from build123d import *

# Parameters (mm, degrees)
ESBO_O1_R                = 2.500003623
ESBO_O1_R_2              = 2.499998411
ESBO_O1_R_3              = 2.500000084
ESBO_O1_R_4              = 2.500000523
ESBO_O1_R_5              = 2.500001341
ESBO_O1_R_6              = 2.499999924
ESBO_O1_R_7              = 2.500000177
ESBO_O1_R_8              = 4
RESSALTO_EXTRUS_O1_DEPTH = 10
ESBO_O2_R                = 4
RESSALTO_EXTRUS_O2_DEPTH = 5


with BuildPart() as part:
    # Esboço1 → Ressalto-extrusão1 (new body)
    with BuildSketch(Plane.XY):
        Polygon((0.059999999, 112.560092658), (0.059999999, -47.439905629), (-39.939999107, -47.439905629), (-59.93999866, -27.439906076), (-59.93999866, 92.560094967), (-39.94000097, 112.560092658), align=None)
        with Locations((-9.939999778, 102.560092881)):
            Circle(ESBO_O1_R, mode=Mode.SUBTRACT)
        with Locations((-9.939999778, 67.560092732)):
            Circle(ESBO_O1_R_2, mode=Mode.SUBTRACT)
        with Locations((-9.939999778, 32.560099544)):
            Circle(ESBO_O1_R_3, mode=Mode.SUBTRACT)
        with Locations((-39.939999107, 51.060092822)):
            Circle(ESBO_O1_R_4, mode=Mode.SUBTRACT)
        with Locations((-39.939999107, 14.06009607)):
            Circle(ESBO_O1_R_5, mode=Mode.SUBTRACT)
        with Locations((-9.939997915, -2.439905703)):
            Circle(ESBO_O1_R_6, mode=Mode.SUBTRACT)
        with Locations((-9.939997915, -37.439905619)):
            Circle(ESBO_O1_R_7, mode=Mode.SUBTRACT)
        with Locations((-39.939999107, -27.93990393)):
            Circle(ESBO_O1_R_8, mode=Mode.SUBTRACT)
        with Locations((-39.94001777, 93.060093764)):
            Circle(ESBO_O1_R_8, mode=Mode.SUBTRACT)
    extrude(amount=RESSALTO_EXTRUS_O1_DEPTH)

    # Esboço2 → Ressalto-extrusão2 (add)
    with BuildSketch(Plane(origin=(0, 0, 0), x_dir=(-1, 0, 0), z_dir=(0, 0, -1))):
        with Locations((39.94001777, 93.060093764)):
            Circle(ESBO_O2_R)
        with Locations((39.939999107, -27.93990393)):
            Circle(ESBO_O2_R)
    extrude(amount=-RESSALTO_EXTRUS_O2_DEPTH)


solid = part.part
Read the model definition and answer for the solid it produces. Units are mm, in the model's axes. A direction names the side the tool comes from. Round coordinates to 2 decimals unless told otherwise and drop trailing zeros. Write each loop counter-clockwise with the first axis right and the second up, starting at its lowest first coordinate (ties: lowest second). Pieces come first, ordered by that corner, then holes.
Q1. Find section A-A on x = -9.94. Determine the outline of the cut face in (y, z).
Values:
outline: (-47.44, 0) - (-39.94, 0) - (-39.94, 10) - (-47.44, 10) - close; (-34.94, 0) - (-4.94, 0) - (-4.94, 10) - (-34.94, 10) - close; (0.06, 0) - (30.06, 0) - (30.06, 10) - (0.06, 10) - close; (35.06, 0) - (65.06, 0) - (65.06, 10) - (35.06, 10) - close; (70.06, 0) - (100.06, 0) - (100.06, 10) - (70.06, 10) - close; (105.06, 0) - (112.56, 0) - (112.56, 10) - (105.06, 10) - close
Q2. A tool of negligible diameter and unlimited length cuts with its end or side. For faces 5 (the face through (-37.79, -24.567, 7.465)), 6 (the face through (-8.6, 34.67, 4.93)), from which of +Z, -Z, +X, -X, +Y, -Y can it reach the whole face along a straight path? Write none if from no direction.
Values:
face 5: +Z
face 6: +Z, -Z
Q3. Flat-ended cylindrical pins translate along their axes: P1, Ø3, axis at x = -9.94, y = 67.56, coming from the +Z side; P2, Ø8, axis at x = -9.94, y = -37.44, coming from the +Z side; P3, Ø2.5, axis at x = -38, y = 92, coming from the +Z side. Find the tip coordinate at first contact, or state that the pin passes through.
Values:
P1: passes through
P2: stops at z = 10
P3: stops at z = 5
Q4. Find section B-B on z = 7.25. State how many separate pieces and enclosed holes the cut face has, and give its area (3 significant figures).
Values:
separate pieces: 1
enclosed holes: 9
area: 8,960 mm2
Q5. The mould has two halves that part along Y. Classify faces 1 (the face through (-20, -47.44, 5)), 2 (the face through (-40, 93, 5)), 3 (the face through (-30, 34, 10)), 4 (the face through (-50.1, 102.4, 4.9)): released by +Y, released by -Y, zero draft, split by the parting line, or undercut.
Values:
face 1: released by -Y
face 2: undercut
face 3: zero draft
face 4: released by +Y
Q6. Find section C-C on x = -49. Determine the outline of the cut face in (y, z), and give its area (3 significant figures).
Values:
outline: (-38.38, 0) - (103.5, 0) - (103.5, 10) - (-38.38, 10) - close
area: 1,420 mm2
Q7. Straight lines are drawn through the part: line 1 (Y direction, x = -9.94, z = 5.75); line 2 (Y direction, x = -10.5, z = 9.75); line 3 (X direction, y = 90, z = 8.75). For each, find the intervals that lie inside material, in ascending order.
Values:
line 1: y = -47.44 to -39.94, -34.94 to -4.94, 0.06 to 30.06, 35.06 to 65.06, 70.06 to 100.06, 105.06 to 112.56
line 2: y = -47.44 to -39.88, -35 to -4.88, 0 to 30.12, 35 to 65.12, 70 to 100.12, 105 to 112.56
line 3: x = -59.94 to -42.52, -37.36 to 0.06
